Read the model definition and answer for the solid it produces. Units are mm, in the model's axes. A direction names the side the tool comes from. Coordinates: 2 decimals unless noted, no trailing zeros. Order: outer loops, then holes, each group sorted by start corner. A loop starts at its lowest first (then second) coordinate and runs counter-clockwise, first axis right, second up. Notation, with made-up numbers: M 27.25,-6 L 82.25,-6 A23 cw 82.25,19 Z; hole C 74.5,52 d3. An arc over 180 degrees is marked long. Write each question's results on one line, items separated by ' | '.
```python
from build123d import *

# Parameters (mm, degrees)
F1_DEPTH = 25


with BuildPart() as f1:
    # F0 (on Front) → F1 (new body)
    with BuildSketch(Plane.XZ):
        with BuildLine():
            Line((-16.52818, 25.036359), (-14.190494, 20.582271))
            ThreePointArc((-14.190494, 20.582271), (-16.578066, 18.712769), (-18.721728, 16.567948))
            Line((-18.721728, 16.567948), (-22.861564, 19.42547))
            ThreePointArc((-22.861564, 19.42547), (-24.689516, 17.041942), (-26.269952, 14.487567))
            Line((-26.269952, 14.487567), (-22.130117, 11.630045))
            ThreePointArc((-22.130117, 11.630045), (-23.375406, 8.865122), (-24.276776, 5.969768))
            Line((-24.276776, 5.969768), (-29.270376, 6.576101))
            ThreePointArc((-29.270376, 6.576101), (-29.781266, 3.6161), (-29.993596, 0.619848))
            Line((-29.993596, 0.619848), (-24.999996, 0.013515))
            ThreePointArc((-24.999996, 0.013515), (-24.817722, -3.013417), (-24.270308, -5.996013))
            Line((-24.270308, -5.996013), (-28.973697, -7.779774))
            ThreePointArc((-28.973697, -7.779774), (-28.050487, -10.638147), (-26.846068, -13.389871))
            Line((-26.846068, -13.389871), (-22.142678, -11.606111))
            ThreePointArc((-22.142678, -11.606111), (-20.574597, -14.201619), (-18.703804, -16.58818))
            Line((-18.703804, -16.58818), (-22.039494, -20.353396))
            ThreePointArc((-22.039494, -20.353396), (-19.89368, -22.455322), (-17.548429, -24.332132))
            Line((-17.548429, -24.332132), (-14.212739, -20.566916))
            ThreePointArc((-14.212739, -20.566916), (-11.618079, -22.136401), (-8.852484, -23.380195))
            Line((-8.852484, -23.380195), (-10.056308, -28.2643))
            ThreePointArc((-10.056308, -28.2643), (-7.17947, -29.128255), (-4.230657, -29.700194))
            Line((-4.230657, -29.700194), (-3.026833, -24.816089))
            ThreePointArc((-3.026833, -24.816089), (0, -25), (3.026833, -24.816089))
            Line((3.026833, -24.816089), (4.230657, -29.700194))
            ThreePointArc((4.230657, -29.700194), (7.17947, -29.128255), (10.056308, -28.2643))
            Line((10.056308, -28.2643), (8.852484, -23.380195))
            ThreePointArc((8.852484, -23.380195), (11.618079, -22.136401), (14.212739, -20.566916))
            Line((14.212739, -20.566916), (17.548429, -24.332132))
            ThreePointArc((17.548429, -24.332132), (19.89368, -22.455322), (22.039494, -20.353396))
            Line((22.039494, -20.353396), (18.703804, -16.58818))
            ThreePointArc((18.703804, -16.58818), (20.574597, -14.201619), (22.142678, -11.606111))
            Line((22.142678, -11.606111), (26.846068, -13.389871))
            ThreePointArc((26.846068, -13.389871), (28.050487, -10.638147), (28.973697, -7.779774))
            Line((28.973697, -7.779774), (24.270308, -5.996013))
            ThreePointArc((24.270308, -5.996013), (24.817722, -3.013417), (24.999996, 0.013515))
            Line((24.999996, 0.013515), (29.993596, 0.619848))
            ThreePointArc((29.993596, 0.619848), (29.781266, 3.6161), (29.270376, 6.576101))
            Line((29.270376, 6.576101), (24.276776, 5.969768))
            ThreePointArc((24.276776, 5.969768), (23.375406, 8.865122), (22.130117, 11.630045))
            Line((22.130117, 11.630045), (26.269952, 14.487567))
            ThreePointArc((26.269952, 14.487567), (24.689516, 17.041942), (22.861564, 19.42547))
            Line((22.861564, 19.42547), (18.721728, 16.567948))
            ThreePointArc((18.721728, 16.567948), (16.578066, 18.712769), (14.190494, 20.582271))
            Line((14.190494, 20.582271), (16.52818, 25.036359))
            ThreePointArc((16.52818, 25.036359), (13.941695, 26.563681), (11.215443, 27.824698))
            Line((11.215443, 27.824698), (8.877758, 23.37061))
            ThreePointArc((8.877758, 23.37061), (5.982892, 24.273545), (3, 24.819347))
            Line((3, 24.819347), (3, 29.849623))
            ThreePointArc((3, 29.849623), (0, 30), (-3, 29.849623))
            Line((-3, 29.849623), (-3, 24.819347))
            ThreePointArc((-3, 24.819347), (-5.982892, 24.273545), (-8.877758, 23.37061))
            Line((-8.877758, 23.37061), (-11.215443, 27.824698))
            ThreePointArc((-11.215443, 27.824698), (-13.941695, 26.563681), (-16.52818, 25.036359))
        make_face()
        with BuildLine():
            ThreePointArc((-5.937197, 4.582543), (-5.303301, 5.303301), (-4.582543, 5.937197))
            Line((-4.582543, 5.937197), (-5.338161, 7.245967))
            ThreePointArc((-5.338161, 7.245967), (-4.5, 7.794229), (-3.606111, 8.245967))
            Line((-3.606111, 8.245967), (-2.850492, 6.937197))
            ThreePointArc((-2.850492, 6.937197), (-1.941143, 7.244444), (-1, 7.433034))
            Line((-1, 7.433034), (-1, 8.944272))
            ThreePointArc((-1, 8.944272), (0, 9), (1, 8.944272))
            Line((1, 8.944272), (1, 7.433034))
            ThreePointArc((1, 7.433034), (1.941143, 7.244444), (2.850492, 6.937197))
            Line((2.850492, 6.937197), (3.606111, 8.245967))
            ThreePointArc((3.606111, 8.245967), (4.5, 7.794229), (5.338161, 7.245967))
            Line((5.338161, 7.245967), (4.582543, 5.937197))
            ThreePointArc((4.582543, 5.937197), (5.303301, 5.303301), (5.937197, 4.582543))
            Line((5.937197, 4.582543), (7.245967, 5.338161))
            ThreePointArc((7.245967, 5.338161), (7.794229, 4.5), (8.245967, 3.606111))
            Line((8.245967, 3.606111), (6.937197, 2.850492))
            ThreePointArc((6.937197, 2.850492), (7.244444, 1.941143), (7.433034, 1))
            Line((7.433034, 1), (8.944272, 1))
            ThreePointArc((8.944272, 1), (9, 0), (8.944272, -1))
            Line((8.944272, -1), (7.433034, -1))
            ThreePointArc((7.433034, -1), (7.244444, -1.941143), (6.937197, -2.850492))
            Line((6.937197, -2.850492), (8.245967, -3.606111))
            ThreePointArc((8.245967, -3.606111), (7.794229, -4.5), (7.245967, -5.338161))
            Line((7.245967, -5.338161), (5.937197, -4.582543))
            ThreePointArc((5.937197, -4.582543), (5.303301, -5.303301), (4.582543, -5.937197))
            Line((4.582543, -5.937197), (5.338161, -7.245967))
            ThreePointArc((5.338161, -7.245967), (4.5, -7.794229), (3.606111, -8.245967))
            Line((3.606111, -8.245967), (2.850492, -6.937197))
            ThreePointArc((2.850492, -6.937197), (1.941143, -7.244444), (1, -7.433034))
            Line((1, -7.433034), (1, -8.944272))
            ThreePointArc((1, -8.944272), (0, -9), (-1, -8.944272))
            Line((-1, -8.944272), (-1, -7.433034))
            ThreePointArc((-1, -7.433034), (-1.941143, -7.244444), (-2.850492, -6.937197))
            Line((-2.850492, -6.937197), (-3.606111, -8.245967))
            ThreePointArc((-3.606111, -8.245967), (-4.5, -7.794229), (-5.338161, -7.245967))
            Line((-5.338161, -7.245967), (-4.582543, -5.937197))
            ThreePointArc((-4.582543, -5.937197), (-5.303301, -5.303301), (-5.937197, -4.582543))
            Line((-5.937197, -4.582543), (-7.245967, -5.338161))
            ThreePointArc((-7.245967, -5.338161), (-7.794229, -4.5), (-8.245967, -3.606111))
            Line((-8.245967, -3.606111), (-6.937197, -2.850492))
            ThreePointArc((-6.937197, -2.850492), (-7.244444, -1.941143), (-7.433034, -1))
            Line((-7.433034, -1), (-8.944272, -1))
            ThreePointArc((-8.944272, -1), (-9, 0), (-8.944272, 1))
            Line((-8.944272, 1), (-7.433034, 1))
            ThreePointArc((-7.433034, 1), (-7.244444, 1.941143), (-6.937197, 2.850492))
            Line((-6.937197, 2.850492), (-8.245967, 3.606111))
            ThreePointArc((-8.245967, 3.606111), (-7.794229, 4.5), (-7.245967, 5.338161))
            Line((-7.245967, 5.338161), (-5.937197, 4.582543))
        make_face(mode=Mode.SUBTRACT)
    extrude(amount=F1_DEPTH)


solid = f1.part
```
(1) The part is cut by section A-A, the plane z = 18.5. Write down the section's boundary in (x, y).
Conclusion:
outline: M -23.62,-25 L -21.52,-25 L -21.52,0 L -23.62,0 Z; M -16.82,-25 L 16.82,-25 L 16.82,0 L -16.82,0 Z; M 21.52,-25 L 23.62,-25 L 23.62,0 L 21.52,0 Z
(2) The part is cut by section C-C, the plane x = -2. Write down the section's boundary in (y, z), then the cut area to 3 significant figures.
Conclusion:
outline: M -25,-24.92 L 0,-24.92 L 0,-7.23 L -25,-7.23 Z; M -25,7.23 L 0,7.23 L 0,29.93 L -25,29.93 Z | area: 1,010 mm²
(3) The part is cut by section D-D, the plane x = 13. Write down the section's boundary in (y, z).
Conclusion:
outline: M -25,-21.35 L 0,-21.35 L 0,27.04 L -25,27.04 Z
(4) The part is cut by section B-B, the plane x = 19.5. Write down the section's boundary in (y, z).
Conclusion:
outline: M -25,-22.8 L 0,-22.8 L 0,-17.49 L -25,-17.49 Z; M -25,-15.64 L 0,-15.64 L 0,17.11 L -25,17.11 Z
(5) For faces 1 (the cylindrical face through (-1.928, -12.325, -7.248)), 2 (the flat face through (3, -12, 27)), 3 (the cylindrical face through (-28.065, -12.325, -10.599)), 4 (the cylindrical face through (-24.823, -12.325, -2.971)), 5 (the flat face through (15.343, -12.325, 22.778)), determine the directions among +Z, -Z, +X, -X, +Y, -Y from which every point of the face is accessible in a straight line to the end or side of a thin tool.
Conclusion:
face 1: +Y, -Y | face 2: +Z, +Y, -Y | face 3: -Z, -X, +Y, -Y | face 4: -X, +Y, -Y | face 5: +X, +Y, -Y
(6) Given pin 1 (0.8 mm diameter, centred on y = -17.5, z = -8.5, fed in from +X); pin 2 (1 mm diameter, centred on y = -11.5, z = 22.5, fed in from +X); pin 3 (1.7 mm diameter, centred on x = -8.5, y = -14, fed in from -Z), each flat-ended and moving along its own axis, determine where each tip first touches the part or whether it passes through.
Conclusion:
pin 1: x = 28.89 | pin 2: x = 15.46 | pin 3: z = -29.01
(7) Straight lines are drawn through the part: line 1 (X direction, y = -13.25, z = -8); line 2 (Z direction, x = -25.5, y = -2); line 3 (Z direction, x = -19, y = -8). For each, find the intervals that lie inside material, in ascending order.
Conclusion:
line 1: -28.91 to -4.12, -3.46 to -1, 1 to 3.46, 4.12 to 28.91 | line 2: -12.88 to -6.46, 0.07 to 6.12, 13.96 to 15.8 | line 3: -23.22 to -16.92, -16.25 to 16.76
(8) The mould has two halves that part along X. Classify faces 6 (the flat face through (-3.637, -12.325, -27.292)), 7 (the flat face through (26.65, -12.32, -6.9)), 8 (the cylindrical face through (-29.776, -12.325, 3.658)): pulls with the +X half, pulls with the -X half, needs draft (parallel to the pull), parting line crosses it, or undercut.
Conclusion:
face 6: undercut | face 7: pulls with the +X half | face 8: pulls with the -X half
